```python
from build123d import *

# Parameters (mm, degrees)
SKETCH_1_W          = 8
SKETCH_1_H          = 10
EXTRUDE_1_DEPTH     = 40
SKETCH_5_W          = 8
SKETCH_5_H          = 10
EXTRUDE_2_DEPTH     = 10
SKETCH_7_R          = 1.6
CUT_EXTRUDE_4_DEPTH = 9
CUT_EXTRUDE_6_DEPTH = 9
SKETCH_3_R          = 1.6
CUT_EXTRUDE_7_DEPTH = 11


with BuildPart() as part:
    # 草图1 → 凸台-拉伸1 (new body)
    with BuildSketch(Plane.XY):
        with Locations((4, 5)):
            Rectangle(SKETCH_1_W, SKETCH_1_H)
    extrude(amount=EXTRUDE_1_DEPTH)

    # 草图5 → 凸台-拉伸2 (add)
    with BuildSketch(Plane(origin=(0, 0, 0), x_dir=(-1, 0, 0), z_dir=(0, 0, -1))):
        with Locations((-4, 5)):
            Rectangle(SKETCH_5_W, SKETCH_5_H)
    extrude(amount=EXTRUDE_2_DEPTH)

    # 草图7 → 切除-拉伸4 (cut, through all)
    with BuildSketch(Plane(origin=(8, 0, 0), x_dir=(0, 0, -1), z_dir=(1, 0, 0))):
        with Locations((7.0094551, 5)):
            Circle(SKETCH_7_R)
    extrude(amount=-CUT_EXTRUDE_4_DEPTH, mode=Mode.SUBTRACT)

    # 草图10 → 切除-拉伸6 (cut, through all)
    with BuildSketch(Plane.ZY):
        with BuildLine():
            Line((40, 5), (40, 5.5))
            Line((40, 5.5), (34.59, 5.5))
            ThreePointArc((34.59, 5.5), (29.63950005, 5), (34.59, 4.5))
            Line((34.59, 4.5), (40, 4.5))
            Line((40, 4.5), (40, 5))
        make_face()
    extrude(amount=-CUT_EXTRUDE_6_DEPTH, mode=Mode.SUBTRACT)

    # 草图3 → 切除-拉伸7 (cut, through all)
    with BuildSketch(Plane.XZ):
        with Locations((4, 37)):
            Circle(SKETCH_3_R)
    extrude(amount=-CUT_EXTRUDE_7_DEPTH, mode=Mode.SUBTRACT)


solid = part.part
```
Check sheet for the modelled part. Datum: model origin and axes. Units: mm. A direction names the side the tool comes from. Round coordinates to 2 decimals unless told otherwise and drop trailing zeros. Order: outer loops, then holes, each group sorted by start corner. A loop starts at its lowest first (then second) coordinate and runs counter-clockwise, first axis right, second up. Notation, with made-up numbers: (-36, 3.25) -> (-14, 3.25) arc R13 ccw to (-14, 28.25) -> close; hole circle Ø10 at (-20.5, -5.75). An arc over 180 degrees is marked (long way). Use CSV: the item, a comma, the result in double quotes.
(1) Cross-section at A-A (x = 4). Record the boundary of the cut face in (y, z).
Worked out:
outline,"(0, -10) -> (10, -10) -> (10, 35.4) -> (5.5, 35.4) -> (5.5, 34.59) arc R2.5 cw (long way) to (4.5, 34.59) -> (4.5, 35.4) -> (0, 35.4) -> close; (0, 38.6) -> (4.5, 38.6) -> (4.5, 40) -> (0, 40) -> close; (5.5, 38.6) -> (10, 38.6) -> (10, 40) -> (5.5, 40) -> close; hole circle Ø3.2 at (5, -7.01)"
(2) Cross-section at D-D (x = 1.75). Record the boundary of the cut face in (y, z), and give its area (3 significant figures).
Worked out:
outline,"(0, -10) -> (10, -10) -> (10, 40) -> (5.5, 40) -> (5.5, 34.59) arc R2.5 cw (long way) to (4.5, 34.59) -> (4.5, 40) -> (0, 40) -> close; hole circle Ø3.2 at (5, -7.01)"
area,"467 mm²"
(3) Tool access check on faces 4 (the face through (4, 5, -10)), 5 (the face through (5, 5.5, 39)). Record the directions out of +Z, -Z, +X, -X, +Y, -Y that give a thin tool (end or side, any length) a straight path to the whole face; none if there is none.
Worked out:
face 4,"-Z, +X, -X, +Y, -Y"
face 5,"+Z, +X, -X"
(4) Cross-section at B-B (z = 32.14). Record the boundary of the cut face in (x, y).
Worked out:
outline,"(0, 0) -> (8, 0) -> (8, 2.5) -> (0, 2.5) -> close; (0, 7.5) -> (8, 7.5) -> (8, 10) -> (0, 10) -> close"
(5) Draft check along Y on faces 1 (the face through (4, 4.5, 39)), 2 (the face through (4, 10, 15)), 3 (the face through (4, 8, 40)). Enter one of: pulls with the +Y half, pulls with the -Y half, needs draft (parallel to the pull), parting line crosses it, or undercut.
Worked out:
face 1,"undercut"
face 2,"pulls with the +Y half"
face 3,"needs draft"
(6) Material ranges on line 1 along Y through (x, z) = (5.75, 37); line 2 along Z through (x, y) = (4, 1.15); line 3 along Z through (x, y) = (4, 3.1), recorded low to high. Write a range as from..to.
Worked out:
line 1,"0..4.5, 5.5..10"
line 2,"-10..35.4, 38.6..40"
line 3,"-10..30.51, 33.77..35.4, 38.6..40"
(7) Cross-section at C-C (y = 5). Record the boundary of the cut face in (x, z), and give its area (3 significant figures).
Worked out:
outline,"(0, -10) -> (8, -10) -> (8, -8.61) -> (0, -8.61) -> close; (0, -5.41) -> (8, -5.41) -> (8, 29.64) -> (0, 29.64) -> close"
area,"292 mm²"
